Verification items for the finished model (mm, model axes). A direction names the side the tool comes from. Coordinates: 2 decimals unless noted, no trailing zeros. Order: outer loops, then holes, each group sorted by start corner. A loop starts at its lowest first (then second) coordinate and runs counter-clockwise, first axis right, second up. Notation, with made-up numbers: M 4,-5.5 L 47,-5.5 A15 ccw 47,20.5 Z; hole C -35.5,-18.75 d7. An arc over 180 degrees is marked long. Return JSON: item names as keys, results as strings. Group by question number.
1. Material ranges on line 1 along X through (y, z) = (-7, -1.5); line 2 along Z through (x, y) = (-21, -13.75); line 3 along X through (y, z) = (-1.25, -2), recorded low to high.
2. Mould release check, pull along Z, two halves, no side actions. Record for faces 3 (the cylindrical face through (0.14, -13.39, 30.65)), 4 (the cylindrical face through (-29.267, -14.148, 28.857)), 5 (the flat face through (0, 0, 0)): +Z half, -Z half, draft (parallel to the pull), parting line (faces both ways), or undercut.
3. Set-up check for faces 1 (the cylindrical face through (30.65, -13.39, -0.14)), 2 (the cylindrical face through (-24.886, -9.39, 0.279)): record each of +Z, -Z, +X, -X, +Y, -Y from which the full face is reachable in a straight line by a thin tool's end or side.
4. Gauge pin test, flat ends, axial feed: pin 1 (5.5 mm diameter, centred on x = 20, z = 0, fed in from -Y); pin 2 (4 mm diameter, centred on x = -11.5, z = 13.5, fed in from -Y); pin 3 (6 mm diameter, centred on y = -17.5, z = -6.5, fed in from -X). Record the tip position at first contact, or that the pin passes through.
5. Section check B-B, the plane z = 0. Record the cut outline in (x, y), plus the area to 3 significant figures.
6. Section check A-A, the plane y = -5.75. Record the cut outline in (x, z).
```python
from build123d import *

# Parameters (mm, degrees)
F1_DEPTH = 1
F3_DEPTH = 26.67
F4_R     = 6.35
F5_DEPTH = 17.78
F6_SIZE  = 0.762
F7_SIZE  = 0.508


with BuildPart() as f1:
    # F0 (on Front) → F1 (new body)
    with BuildSketch(Plane.XZ):
        with BuildLine():
            ThreePointArc((-9.251368, 33.047819), (-30.124369, 30.124369), (-33.047819, 9.251368))
            ThreePointArc((-33.047819, 9.251368), (-30.650587, 0), (-33.047819, -9.251368))
            ThreePointArc((-33.047819, -9.251368), (-30.124369, -30.124369), (-9.251368, -33.047819))
            ThreePointArc((-9.251368, -33.047819), (0, -30.650587), (9.251368, -33.047819))
            ThreePointArc((9.251368, -33.047819), (30.124369, -30.124369), (33.047819, -9.251368))
            ThreePointArc((33.047819, -9.251368), (30.650587, 0), (33.047819, 9.251368))
            ThreePointArc((33.047819, 9.251368), (30.124369, 30.124369), (9.251368, 33.047819))
            ThreePointArc((9.251368, 33.047819), (0, 30.650587), (-9.251368, 33.047819))
        make_face()
    extrude(amount=F1_DEPTH)

    # F2 (on face) → F3 (join)
    with BuildSketch(Plane.XZ.offset(1)):
        with BuildLine():
            ThreePointArc((-9.251368, 33.047819), (-30.124369, 30.124369), (-33.047819, 9.251368))
            ThreePointArc((-33.047819, 9.251368), (-30.650587, 0), (-33.047819, -9.251368))
            ThreePointArc((-33.047819, -9.251368), (-30.124369, -30.124369), (-9.251368, -33.047819))
            ThreePointArc((-9.251368, -33.047819), (0, -30.650587), (9.251368, -33.047819))
            ThreePointArc((9.251368, -33.047819), (30.124369, -30.124369), (33.047819, -9.251368))
            ThreePointArc((33.047819, -9.251368), (30.650587, 0), (33.047819, 9.251368))
            ThreePointArc((33.047819, 9.251368), (30.124369, 30.124369), (9.251368, 33.047819))
            ThreePointArc((9.251368, 33.047819), (0, 30.650587), (-9.251368, 33.047819))
        make_face()
        with BuildLine():
            ThreePointArc((-9.979822, 31.736577), (0, 29.150587), (9.979822, 31.736577))
            ThreePointArc((9.979822, 31.736577), (29.063708, 29.063708), (31.736577, 9.979822))
            ThreePointArc((31.736577, 9.979822), (29.150587, 0), (31.736577, -9.979822))
            ThreePointArc((31.736577, -9.979822), (29.063708, -29.063708), (9.979822, -31.736577))
            ThreePointArc((9.979822, -31.736577), (0, -29.150587), (-9.979822, -31.736577))
            ThreePointArc((-9.979822, -31.736577), (-29.063708, -29.063708), (-31.736577, -9.979822))
            ThreePointArc((-31.736577, -9.979822), (-29.150587, 0), (-31.736577, 9.979822))
            ThreePointArc((-31.736577, 9.979822), (-29.063708, 29.063708), (-9.979822, 31.736577))
        make_face(mode=Mode.SUBTRACT)
    extrude(amount=F3_DEPTH)

    # F4 (on face) → F5 (join)
    with BuildSketch(Plane.XZ.offset(1)):
        with Locations((-18.542, 0)):
            Circle(F4_R)
        with Locations((18.542, 0)):
            Circle(F4_R)
    extrude(amount=F5_DEPTH)

    # F6
    f6_edges = [f1.edges().sort_by_distance(p)[0] for p in [
        (12.192, -18.78, 0),
        (-24.892, -18.78, 0),
    ]]
    chamfer(f6_edges, length=F6_SIZE)

    # F7
    f7_edges = [f1.edges().sort_by_distance(p)[0] for p in [
        (-30.124369, -27.67, 30.124369),
    ]]
    chamfer(f7_edges, length=F7_SIZE)


solid = f1.part
```
Answers follow:
{
 "1": {"line 1": "-30.71 to -29.21, -24.71 to -12.37, 12.37 to 24.71, 29.21 to 30.71", "line 2": "-34.95 to -33.42, -5.85 to 5.85, 33.42 to 34.95", "line 3": "-30.76 to -29.25, -24.57 to -12.52, 12.52 to 24.57, 29.25 to 30.76"},
 "2": {"face 3": "+Z half", "face 4": "undercut", "face 5": "draft"},
 "3": {"face 1": "+X, +Y, -Y", "face 2": "-Y"},
 "4": {"pin 1": "y = -18.78", "pin 2": "y = -1", "pin 3": "x = -33.18"},
 "5": {"outline": "M -30.65,-27.16 L -30.14,-27.67 L -29.15,-27.67 L -29.15,-1 L -24.89,-1 L -24.89,-18.02 L -24.13,-18.78 L -12.95,-18.78 L -12.19,-18.02 L -12.19,-1 L 12.19,-1 L 12.19,-18.02 L 12.95,-18.78 L 24.13,-18.78 L 24.89,-18.02 L 24.89,-1 L 29.15,-1 L 29.15,-27.67 L 30.14,-27.67 L 30.65,-27.16 L 30.65,0 L -30.65,0 Z", "area": "592 mm^2"},
 "6": {"outline": "M -33.05,-9.25 A17.5 ccw -9.25,-33.05 A19.05 cw 9.25,-33.05 A17.5 ccw 33.05,-9.25 A19.05 cw 33.05,9.25 A17.5 ccw 9.25,33.05 A19.05 cw -9.25,33.05 A17.5 ccw -33.05,9.25 A19.05 cw Z; C -18.54,0 d12.7; C 18.54,0 d12.7; hole M -31.74,-9.98 A16 ccw -9.98,-31.74 A20.55 cw 9.98,-31.74 A16 ccw 31.74,-9.98 A20.55 cw 31.74,9.98 A16 ccw 9.98,31.74 A20.55 cw -9.98,31.74 A16 ccw -31.74,9.98 A20.55 cw Z"}
}
